Geometry check sheet. Reference: the model listing, model coordinates, mm. Coordinates: 2 decimals unless noted, no trailing zeros. Order: outer loops, then holes, each group sorted by start corner. A loop starts at its lowest first (then second) coordinate and runs counter-clockwise, first axis right, second up.
```python
from build123d import *

# Parameters (mm, degrees)
F1_DEPTH      = 33.782
F1_DEPTH_BACK = 25.4


with BuildPart() as f1:
    # F0 (on Top) → F1 (new body, two sides)
    with BuildSketch(Plane.XY) as f1_sk:
        Polygon((18.1071458891, -27.7275939392), (23.3180151746, -23.5150667919), (27.5742421791, -18.3398300471), (30.7015764689, -12.4137585054), (32.5719846108, -5.979466232), (33.1088918757, 0.6996260916), (32.2903172171, 7.3500756408), (30.1497731777, 13.6996122296), (26.7748938819, 19.4882850841), (22.3038472847, 24.4791052575), (16.9196785591, 28.4677479855), (10.8428162052, 31.2909177661), (4.322047682, 32.8330336969), (-2.3756659812, 33.0309613704), (-8.9761196, 31.8765976044), (-15.2090898277, 29.4172021872), (-20.8193981308, 25.753463056), (-25.5773578283, 21.0353741214), (-29.2881774911, 15.4560944988), (-31.7999357262, 9.2440405513), (-33.0098008564, 2.6535344976), (-32.868240861, -4.0456075703), (-31.3810512229, -10.5791219889), (-28.6091176606, -16.6795259103), (-24.6659234598, -22.0970680811), (-19.7129034545, -26.6099536884), (-13.9528348656, -30.0334246652), (-7.6215355779, -32.2273237074), (-0.9782097282, -33.1018323305), (5.7051641428, -32.6211480486), (12.1549679234, -30.8049501329), align=None)
    extrude(amount=-F1_DEPTH)
    extrude(f1_sk.sketch, amount=F1_DEPTH_BACK)


solid = f1.part
```
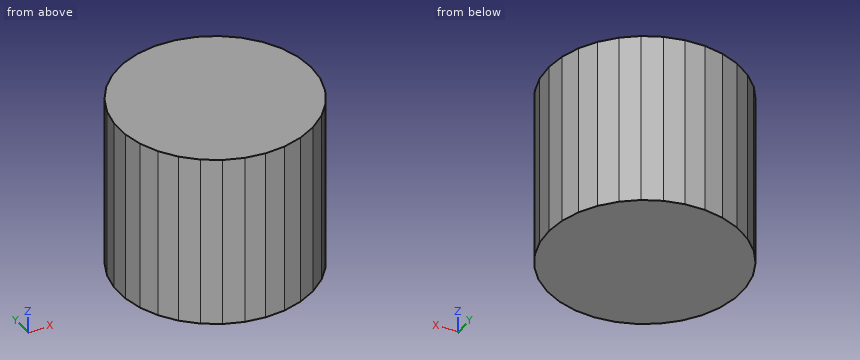
Item 1: Sectioned sample at C-C (y = -20). Record the cut outline in (x, z).
Item 2: Sectioned sample at B-B (x = -27). Record the cut outline in (y, z).
Item 3: Thickness scan on line 1 along X through (y, z) = (19.5, -18); line 2 along X through (y, z) = (-14, 3); line 3 along Y through (x, z) = (-23, -5.5). Record the ranges inside material, lowest first.
Item 4: Depth check by flat-ended pin: P1, Ø8, axis at x = -8.5, z = -14.5, coming from the -Y side; P2, Ø8, axis at y = -17, z = -7.5, coming from the +X side; P3, Ø2, axis at x = 17.5, z = -11.5, coming from the -Y side; P4, Ø1, axis at y = 2.5, z = -20.5, coming from the -X side. Enter the tip coordinate at first touch or a pass-through.
Geometry check:
1. outline: (-26.19, -33.78) - (26.21, -33.78) - (26.21, 25.4) - (-26.19, 25.4) - close
2. outline: (-18.89, -33.78) - (18.9, -33.78) - (18.9, 25.4) - (-18.89, 25.4) - close
3. line 1: x = -26.6 to 26.76
3. line 2: x = -29.83 to 29.86
3. line 3: y = -23.61 to 23.59
4. P1: stops at y = -32.64
4. P2: stops at x = 30.39
4. P3: stops at y = -28.56
4. P4: stops at x = -33.01
